CAD build for the part. Positions are in the model's coordinates, mm. Give positions to 0.01 mm unless a question says otherwise; leave off trailing zeros. Order: outer loops, then holes, each group sorted by start corner. A loop starts at its lowest first (then second) coordinate and runs counter-clockwise, first axis right, second up.
```python
from build123d import *

# Parameters (mm, degrees)
F0_R      = 15
F0_R_2    = 11.5
F1_DEPTH  = 0.8
F0_R_3    = 9.5
F2_DEPTH  = 80
F4_R      = 9.5
F5_DEPTH  = 3
F7_R      = 9.5
F8_DEPTH  = 3
F10_DEPTH = 1
F11_COUNT = 3
F11_ANGLE = 120


with BuildPart() as f1:
    # F0 (on Top) → F1 (new body)
    with BuildSketch(Plane.XY):
        Circle(F0_R)
        Circle(F0_R_2, mode=Mode.SUBTRACT)
    extrude(amount=F1_DEPTH)



with BuildPart() as f1b:
    # F0 (on Top) → F1, piece 2 (new body)
    with BuildSketch(Plane.XY):
        Circle(F0_R_3)
    extrude(amount=F1_DEPTH)


with BuildPart() as f1_1:
    add(f1.part)

    add(f1b.part)  # F2 merges F1b
    # F0 (on Top) → F2 (join)
    with BuildSketch(Plane.XY):
        Circle(F0_R_2)
        Circle(F0_R_3, mode=Mode.SUBTRACT)
    extrude(amount=F2_DEPTH)

    # F4 (on offset) → F5 (join)
    with BuildSketch(Plane.XY.offset(20.8)):
        Circle(F4_R)
    extrude(amount=F5_DEPTH)

    # F7 (on offset) → F8 (join)
    with BuildSketch(Plane.XY.offset(58.8)):
        Circle(F7_R)
    extrude(amount=-F8_DEPTH)

    # F9 (on Front) → F10 (join, symmetric)
    with BuildSketch(Plane.XZ):
        Polygon((-1, 20.8), (-9.5, 20.8), (-9.5, 10.7640403081), (-2.1869234638, 19.3985981129), align=None)
        Polygon((0, 20.8), (-1, 20.8), (-2.1869234638, 19.3985981129), (0, 19.3985981129), (2.1869234638, 19.3985981129), (1, 20.8), align=None)
        Polygon((9.5, 20.8), (1, 20.8), (2.1869234638, 19.3985981129), (9.5, 10.7640403081), align=None)
        Polygon((-1.3762295453, 55.4016393049), (-1, 55.8), (-9.5, 55.8), (-9.5, 46.8), align=None)
        Polygon((0, 55.8), (-1, 55.8), (-1.3762295453, 55.4016393049), (0, 55.4016393049), (1.3762295453, 55.4016393049), (1, 55.8), align=None)
        Polygon((9.5, 55.8), (1, 55.8), (1.3762295453, 55.4016393049), (9.5, 46.8), align=None)
    extrude(amount=F10_DEPTH, both=True)

    # F11: F1 ×3 about axis
    f11_axis = Axis((0, 0, 50), (0, 0, 1))


with BuildPart() as f1_2:
    add(f1_1.part)
    for i in range(1, F11_COUNT):
        add(f1_1.part.rotate(f11_axis, i * F11_ANGLE / (F11_COUNT - 1)))


solid = f1_2.part
```
Item 1: Wall check: L1, parallel to Z at x = 1.5, y = 7.75; L2, parallel to Y at x = 0, z = 64.5. Give the ranges that are in metal, low to high.
Item 2: Slice it at A-A (y = 0). Give the cut face in (x, z), and give its area (3 significant figures).
Item 3: Slice it at D-D (x = -10.75). Give the cut face in (y, z), and give its area (3 significant figures).
Item 4: Slice it at C-C (z = 30). Give the cut face in (x, y).
Item 5: Two-plate mould, pull along Z, no slides. Class faces 1 (the face through (-1.5, 11.4, 39.8)), 2 (the face through (5.38, -0.01, 51.16)), 3 (the face through (4.062, 5.036, 52.384)): released by +Z, released by -Z, zero draft, split by the parting line, or undercut.
Item 6: Drop flat-ended pins along their axis: pin 1 Ø5 at (x, z) = (-5, 67) entering from +Y (3 decimals); pin 2 Ø5 at (x, y) = (10.5, 5) entering from -Z; pin 3 Ø8 at (y, z) = (-10.5, 65.5) entering from -X; pin 4 Ø17 at (x, y) = (0, 0) entering from +Z. Give the stop position or say it passes through.
Item 7: Slice it at B-B (x = 8.25). Give the cut face in (y, z).
A:
1. L1: z = 0 to 0.8, 20.8 to 23.8, 55.8 to 58.8
1. L2: y = -11.5 to -9.5, 9.5 to 11.5
2. outline: (-15, 0) - (15, 0) - (15, 0.8) - (11.5, 0.8) - (11.5, 80) - (9.5, 80) - (9.5, 58.8) - (-9.5, 58.8) - (-9.5, 80) - (-11.5, 80) - (-11.5, 0.8) - (-15, 0.8) - close; hole (-9.5, 0.8) - (9.5, 0.8) - (9.5, 10.76) - (2.19, 19.4) - (-2.19, 19.4) - (-9.5, 10.76) - close; hole (-9.5, 23.8) - (9.5, 23.8) - (9.5, 46.8) - (1.38, 55.4) - (-1.38, 55.4) - (-9.5, 46.8) - close
2. area: 622 mm2
3. outline: (-10.46, 0) - (10.46, 0) - (10.46, 0.8) - (4.09, 0.8) - (4.09, 80) - (-4.09, 80) - (-4.09, 0.8) - (-10.46, 0.8) - close
3. area: 664 mm2
4. outline: circle Ø23 at (0, 0); hole circle Ø19 at (0, 0)
5. face 1: zero draft
5. face 2: undercut
5. face 3: undercut
6. pin 1: stops at y = 11.225
6. pin 2: stops at z = 0
6. pin 3: stops at x = -9.49
6. pin 4: stops at z = 58.8
7. outline: (-12.53, 0) - (12.53, 0) - (12.53, 0.8) - (8.01, 0.8) - (8.01, 80) - (4.71, 80) - (4.71, 58.8) - (-4.71, 58.8) - (-4.71, 80) - (-8.01, 80) - (-8.01, 0.8) - (-12.53, 0.8) - close; hole (-4.71, 0.8) - (4.71, 0.8) - (4.71, 20.8) - (1, 20.8) - (1, 12.24) - (-1, 12.24) - (-1, 20.8) - (-4.71, 20.8) - close; hole (-4.71, 23.8) - (4.71, 23.8) - (4.71, 55.8) - (1, 55.8) - (1, 48.12) - (-1, 48.12) - (-1, 55.8) - (-4.71, 55.8) - close
